```python
from build123d import *

# Parameters (mm, degrees)
SKETCH1_W           = 210
SKETCH1_H           = 15
BOSS_EXTRUDE1_DEPTH = 5
SKETCH2_W           = 50
SKETCH2_H           = 5
BOSS_EXTRUDE2_DEPTH = 5
SKETCH3_W           = 5
SKETCH3_H           = 7.5
CUT_EXTRUDE1_DEPTH  = 5
BOSS_EXTRUDE3_DEPTH = 5


with BuildPart() as part:
    # Sketch1 → Boss-Extrude1 (new body)
    with BuildSketch(Plane.XY):
        with Locations((-105, 7.5)):
            Rectangle(SKETCH1_W, SKETCH1_H)
    extrude(amount=BOSS_EXTRUDE1_DEPTH)

    # Sketch2 → Boss-Extrude2 (add)
    with BuildSketch(Plane(origin=(0, 0, 0), x_dir=(-1, 0, 0), z_dir=(0, 0, -1))):
        with Locations((45, -2.5)):
            Rectangle(SKETCH2_W, SKETCH2_H)
        with Locations((165, -2.5)):
            Rectangle(SKETCH2_W, SKETCH2_H)
        with Locations((165, 17.5)):
            Rectangle(SKETCH2_W, SKETCH2_H)
        with Locations((45, 17.5)):
            Rectangle(SKETCH2_W, SKETCH2_H)
    extrude(amount=-BOSS_EXTRUDE2_DEPTH)

    # Sketch3 → Cut-Extrude1 (cut)
    with BuildSketch(Plane(origin=(0, 0, 0), x_dir=(-1, 0, 0), z_dir=(0, 0, -1))):
        with Locations((2.5, 3.75)):
            Rectangle(SKETCH3_W, SKETCH3_H)
        with Locations((207.5, 3.75)):
            Rectangle(SKETCH3_W, SKETCH3_H)
    extrude(amount=-CUT_EXTRUDE1_DEPTH, mode=Mode.SUBTRACT)

    # Sketch4 → Boss-Extrude3 (add)
    with BuildSketch(Plane(origin=(0, 0, 0), x_dir=(-1, 0, 0), z_dir=(0, 0, -1))):
        Polygon((140, 30), (140, 20), (145, 20), (145, 25), (185, 25), (185, 20), (190, 20), (190, 30), align=None)
        Polygon((20, 20), (25, 20), (25, 25), (65, 25), (65, 20), (70, 20), (70, 30), (20, 30), align=None)
        Polygon((70, -15), (70, -5), (65, -5), (65, -10), (25, -10), (25, -5), (20, -5), (20, -15), align=None)
        Polygon((190, -5), (185, -5), (185, -10), (145, -10), (145, -5), (140, -5), (140, -15), (190, -15), align=None)
    extrude(amount=-BOSS_EXTRUDE3_DEPTH)


solid = part.part
```
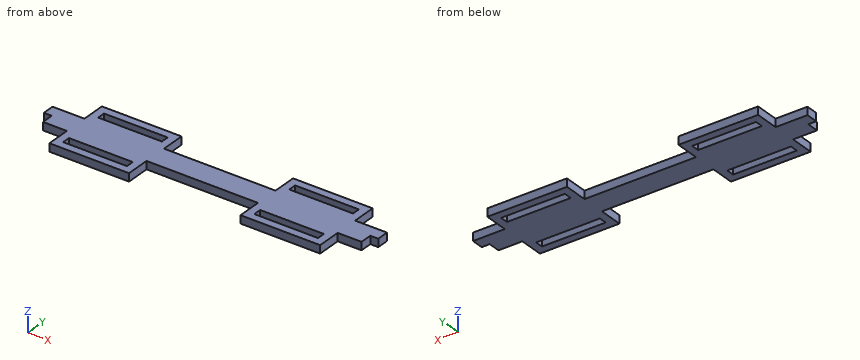
Verification items for the finished model (mm, model axes). Give positions to 0.01 mm unless a question says otherwise; leave off trailing zeros. Order: outer loops, then holes, each group sorted by start corner. A loop starts at its lowest first (then second) coordinate and runs counter-clockwise, first axis right, second up. Notation, with made-up numbers: (38, 49.5) -> (90, 49.5) arc R29 cw to (90, 71.5) -> close; hole circle Ø7 at (11.25, -32). An arc over 180 degrees is marked (long way). Use a Markdown table: item, result.
1) Section check B-B, the plane y = 18. Record the boundary of the cut face in (x, z), then the cut area to 3 significant figures.
Results:
| item | result |
|---|---|
| outline | (-190, 0) -> (-140, 0) -> (-140, 5) -> (-190, 5) -> close; (-70, 0) -> (-20, 0) -> (-20, 5) -> (-70, 5) -> close |
| area | 500 mm² |
2) Material ranges on probe 1 along X at (y, z) = (-9.5, 1.7); probe 2 along Y at (x, z) = (-182.5, 4.15); probe 3 along X at (y, z) = (-3, 4.4), recorded low to high.
Results:
| item | result |
|---|---|
| probe 1 | -190 to -185, -145 to -140, -70 to -65, -25 to -20 |
| probe 2 | -15 to -10, -5 to 20, 25 to 30 |
| probe 3 | -190 to -140, -70 to -20 |
3) Section check C-C, the plane z = 2.45. Give the number of separate pieces and of enclosed holes in the cut face, then the cut area to 4 significant figures.
Results:
| item | result |
|---|---|
| separate pieces | 1 |
| enclosed holes | 4 |
| area | 5,275 mm² |
4) Section check A-A, the plane x = -170.5. Record the boundary of the cut face in (y, z), then the cut area to 3 significant figures.
Results:
| item | result |
|---|---|
| outline | (-15, 0) -> (-10, 0) -> (-10, 5) -> (-15, 5) -> close; (-5, 0) -> (20, 0) -> (20, 5) -> (-5, 5) -> close; (25, 0) -> (30, 0) -> (30, 5) -> (25, 5) -> close |
| area | 175 mm² |
5) Depth check by flat-ended pin: pin 1 Ø2.5 at (y, z) = (20, 2) entering from -X; pin 2 Ø1.5 at (y, z) = (-6.5, 3.5) entering from +X; pin 3 Ø2.5 at (x, z) = (-8, 2) entering from +Y. Enter the tip coordinate at first touch or a pass-through.
Results:
| item | result |
|---|---|
| pin 1 | x = -190 |
| pin 2 | x = -20 |
| pin 3 | y = 15 |
6) Section check D-D, the plane x = -123.5. Record the boundary of the cut face in (y, z).
Results:
| item | result |
|---|---|
| outline | (0, 0) -> (15, 0) -> (15, 5) -> (0, 5) -> close |
